Build history of the part. All positions in model axes, mm. Round coordinates to 2 decimals unless told otherwise and drop trailing zeros. Write each loop counter-clockwise with the first axis right and the second up, starting at its lowest first coordinate (ties: lowest second). Pieces come first, ordered by that corner, then holes. Notation, with made-up numbers: M -35.5,-36 L -7.5,-36 A16 cw -7.5,-28 Z; hole C 83.5,60 d7. An arc over 180 degrees is marked long. Use a Markdown table: item, result.
from build123d import *

# Parameters (mm, degrees)
SKETCH_1_W                  = 35
SKETCH_1_H                  = 35
EXTRUDE_1_DEPTH             = 4.5
CHAMFER_1_SIZE              = 2
PATTERN_LINEAR_1_COUNT      = 2
PATTERN_LINEAR_1_PITCH      = 25
PATTERN_LINEAR_1_COUNT_DIR2 = 2
PATTERN_LINEAR_1_PITCH_DIR2 = 26


with BuildPart() as part:
    # Эскиз1 → Бобышка-Вытянуть1 (new body)
    with BuildSketch(Plane(origin=(0, 0, 0), x_dir=(0, 0, -1), z_dir=(1, 0, 0))):
        Rectangle(SKETCH_1_W, SKETCH_1_H)
    extrude(amount=EXTRUDE_1_DEPTH)

    # Фаска1
    chamfer_1_edges = [part.edges().sort_by_distance(p)[0] for p in [
        (2.25, -17.5, -17.5),
        (2.25, -17.5, 17.5),
        (2.25, 17.5, 17.5),
        (2.25, 17.5, -17.5),
    ]]
    chamfer(chamfer_1_edges, length=CHAMFER_1_SIZE)

    # Эскиз3 → Отверстие с зазором M41 (revolve, cut)
    with BuildSketch(Plane(origin=(4.5, 13, -12.5), x_dir=(0, 0, -1), z_dir=(0, 1, 0))):
        Polygon((0, 0), (0, 21.351936393), (2.25, 20), (2.25, 0), align=None)
    hole_wizard_m41 = revolve(axis=Axis((10.85, 13, -12.5), (-1, 0, 0)), mode=Mode.SUBTRACT)

    # Линейный массив1: Hole Wizard M41 2 × 2
    with Locations(*[(0, -j * PATTERN_LINEAR_1_PITCH_DIR2, i * PATTERN_LINEAR_1_PITCH) for i in range(PATTERN_LINEAR_1_COUNT) for j in range(PATTERN_LINEAR_1_COUNT_DIR2) if (i, j) != (0, 0)]):
        add(hole_wizard_m41, mode=Mode.SUBTRACT)


solid = part.part
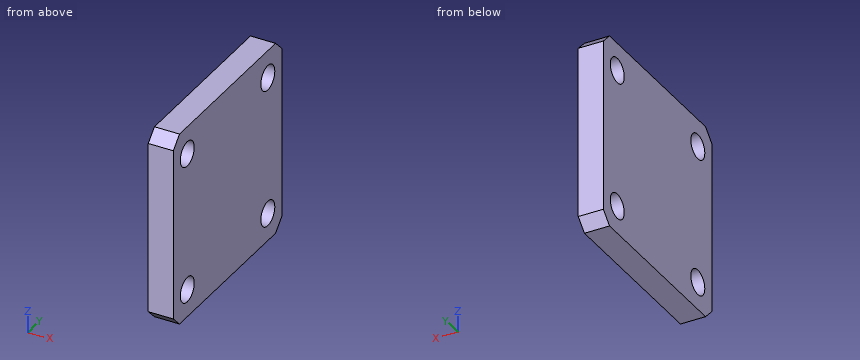
Q1. Cut at C-C on x = 1.85. Give the cut face in (y, z), and give its area (3 significant figures).
Response values:
| item | result |
|---|---|
| outline | M -17.5,-15.5 L -15.5,-17.5 L 15.5,-17.5 L 17.5,-15.5 L 17.5,15.5 L 15.5,17.5 L -15.5,17.5 L -17.5,15.5 Z; hole C -13,-12.5 d4.5; hole C -13,12.5 d4.5; hole C 13,-12.5 d4.5; hole C 13,12.5 d4.5 |
| area | 1,150 mm2 |
Q2. Cut at B-B on z = -12.5. Give the cut face in (x, y).
Response values:
| item | result |
|---|---|
| outline | M 0,-17.5 L 4.5,-17.5 L 4.5,-15.25 L 0,-15.25 Z; M 0,-10.75 L 4.5,-10.75 L 4.5,10.75 L 0,10.75 Z; M 0,15.25 L 4.5,15.25 L 4.5,17.5 L 0,17.5 Z |
Q3. Drill centre lines: L1, parallel to Z at x = 2.6, y = 13; L2, parallel to Y at x = 1.8, z = 12.5; L3, parallel to Z at x = 0.25, y = -11. Where is each one in solid material? Low to high.
Response values:
| item | result |
|---|---|
| L1 | z = -17.5 to -14.75, -10.25 to 10.25, 14.75 to 17.5 |
| L2 | y = -17.5 to -15.25, -10.75 to 10.75, 15.25 to 17.5 |
| L3 | z = -17.5 to -13.53, -11.47 to 11.47, 13.53 to 17.5 |
Q4. Cut at A-A on y = -13. Give the cut face in (x, z), and give its area (3 significant figures).
Response values:
| item | result |
|---|---|
| outline | M 0,-17.5 L 4.5,-17.5 L 4.5,-14.75 L 0,-14.75 Z; M 0,-10.25 L 4.5,-10.25 L 4.5,10.25 L 0,10.25 Z; M 0,14.75 L 4.5,14.75 L 4.5,17.5 L 0,17.5 Z |
| area | 117 mm2 |
Q5. Drop a flat-ended pin along its axis: P1, Ø12, axis at y = -8.5, z = -7, coming from the -X side. Give the stop position or say it passes through.
Response values:
| item | result |
|---|---|
| P1 | stops at x = 0 |
